Work out the finished part from the listing and answer in its coordinate system (mm). A direction names the side the tool comes from. Round coordinates to 2 decimals unless told otherwise and drop trailing zeros. Order: outer loops, then holes, each group sorted by start corner. A loop starts at its lowest first (then second) coordinate and runs counter-clockwise, first axis right, second up.
from build123d import *

# Parameters (mm, degrees)
SKETCH1_R               = 16.63
SKETCH1_R_2             = 4.8
SKETCH1_R_3             = 2.625
BOSS_EXTRUDE2_DEPTH     = 2
SKETCH5_R               = 6.625
SKETCH5_R_2             = 2.625
BOSS_EXTRUDE3_DEPTH     = 8
SKETCH4_R               = 1.6
CUT_EXTRUDE1_DEPTH      = 8
CIRPATTERN1_COUNT       = 2
CUT_EXTRUDE2_DEPTH      = 10
CUT_EXTRUDE2_DEPTH_BACK = 8
SKETCH6_R               = 1.5


with BuildPart() as part:
    # Sketch1 → Boss-Extrude2 (new body)
    # profile 1 of 2: a face of its own
    with BuildSketch(Plane(origin=(0, 0, 0), x_dir=(1, 0, 0), z_dir=(0, 1, 0))):
        with Locations(Location((0, 0, 0), (0, 0, 270))):
            Circle(SKETCH1_R)
        Circle(SKETCH1_R_2, mode=Mode.SUBTRACT)
    # profile 2 of 2: a face of its own
    with BuildSketch(Plane(origin=(0, 0, 0), x_dir=(1, 0, 0), z_dir=(0, 1, 0))):
        Circle(SKETCH1_R_2)
        with Locations(Location((0, 0, 0), (0, 0, 270))):
            Circle(SKETCH1_R_3, mode=Mode.SUBTRACT)
    extrude(amount=BOSS_EXTRUDE2_DEPTH)

    # Sketch5 → Boss-Extrude3 (add)
    with BuildSketch(Plane(origin=(0, 2, 0), x_dir=(1, 0, 0), z_dir=(0, 1, 0))):
        with Locations(Location((0, 0, 0), (0, 0, 270))):
            Circle(SKETCH5_R)
        with Locations(Location((0, 0, 0), (0, 0, 270))):
            Circle(SKETCH5_R_2, mode=Mode.SUBTRACT)
    extrude(amount=BOSS_EXTRUDE3_DEPTH)

    # Sketch4 → Cut-Extrude1 (cut)
    with BuildSketch(Plane(origin=(0, 2, 0), x_dir=(1, 0, 0), z_dir=(0, 1, 0))):
        with Locations(Location((11.625, 0, 0), (0, 0, 270))):
            Circle(SKETCH4_R)
    cut_extrude1 = extrude(amount=-CUT_EXTRUDE1_DEPTH, mode=Mode.SUBTRACT)

    # CirPattern1: Cut-Extrude1 ×2 about axis
    cirpattern1_axis = Axis((0, 0, 0), (0, 1, 0))
    for i in range(1, CIRPATTERN1_COUNT):
        add(cut_extrude1.rotate(cirpattern1_axis, i * 360 / CIRPATTERN1_COUNT), mode=Mode.SUBTRACT)

    # Sketch6 → Cut-Extrude2 (cut, two sides: drawn at the far end of the back side and taken through both)
    with BuildSketch(Plane(origin=(0, 0, 0), x_dir=(0, 0, -1), z_dir=(1, 0, 0)).offset(-CUT_EXTRUDE2_DEPTH_BACK)):
        with Locations(Location((0, 5.866356901, 0), (0, 0, 180))):
            Circle(SKETCH6_R)
    extrude(amount=CUT_EXTRUDE2_DEPTH + CUT_EXTRUDE2_DEPTH_BACK, mode=Mode.SUBTRACT)


solid = part.part
Item 1: Find section B-B (x = 0). Write down the section's boundary in (y, z) (3 decimals).
Item 2: Find the intervals of material crossed by line 1 along X through (y, z) = (0.7, 0) (3 decimals); line 2 along Y through (x, z) = (-5.5, -13.5); line 3 along Z through (x, y) = (-0.5, 9.25), in increasing order.
Item 3: Find section A-A (z = 0). Write down the section's boundary in (x, y) (3 decimals), plus the area to 3 significant figures.
Item 4: Given pin 1 (2.5 mm diameter, centred on y = 5.87, z = 0, fed in from +X); pin 2 (3 mm diameter, centred on y = 8.5, z = -7, fed in from -X); pin 3 (1.5 mm diameter, centred on x = 5, y = 3.5, fed in from -Z); pin 4 (2 mm diameter, centred on x = -5, z = 11, fed in from +Y), each flat-ended and moving along its own axis, determine where each tip first touches the part or whether it passes through.
Item 5: Find section C-C (y = 8). Write down the section's boundary in (x, z) (3 decimals), plus the area to 3 significant figures.
Item 6: A tool of negligible diameter and unlimited length cuts with its end or side. For faces 1 (the face through (4.36, 7.33, -0.33)), 2 (the face through (0, 2, 7)), from which of +Z, -Z, +X, -X, +Y, -Y can it reach the whole face along a straight path? Write none if from no direction.
Item 7: Find section D-D (x = -3.5). Write down the section's boundary in (y, z) (3 decimals).
Item 8: For a pull along Y with two mould halves and no side action, classify faces 3 (the face through (-4.4, 5.8, -1.5)), 4 (the face through (-16.235, 0.986, -3.605)), 5 (the face through (0, 10, 3)), 6 (the face through (0, 0, 3)) as released by +Y, released by -Y, zero draft, split by the parting line, or undercut.
Model answer:
1. outline: (0, -16.63) - (2, -16.63) - (2, -6.625) - (10, -6.625) - (10, -2.625) - (0, -2.625) - close; (0, 2.625) - (10, 2.625) - (10, 6.625) - (2, 6.625) - (2, 16.63) - (0, 16.63) - close
2. line 1: x = -16.63 to -13.225, -10.025 to -2.625, 2.625 to 10.025, 13.225 to 16.63
2. line 2: y = 0 to 2
2. line 3: z = -6.61 to -2.58, 2.58 to 6.61
3. outline: (-16.63, 0) - (-13.225, 0) - (-13.225, 2) - (-16.63, 2) - close; (-10.025, 0) - (-2.625, 0) - (-2.625, 4.366) - (-6.625, 4.366) - (-6.625, 2) - (-10.025, 2) - close; (-6.625, 7.366) - (-2.625, 7.366) - (-2.625, 10) - (-6.625, 10) - close; (2.625, 0) - (10.025, 0) - (10.025, 2) - (6.625, 2) - (6.625, 4.366) - (2.625, 4.366) - close; (2.625, 7.366) - (6.625, 7.366) - (6.625, 10) - (2.625, 10) - close; (13.225, 0) - (16.63, 0) - (16.63, 2) - (13.225, 2) - close
3. area: 83.2 mm2
4. pin 1: passes through
4. pin 2: stops at x = -3.69
4. pin 3: stops at z = -5.08
4. pin 4: stops at y = 2
5. outline: circle Ø13.25 at (0, 0); hole circle Ø5.25 at (0, 0)
5. area: 116 mm2
6. face 1: +X, -X
6. face 2: +Y
7. outline: (0, -16.258) - (2, -16.258) - (2, -5.625) - (10, -5.625) - (10, 5.625) - (2, 5.625) - (2, 16.258) - (0, 16.258) - close; hole circle Ø3 at (5.866, 0)
8. face 3: undercut
8. face 4: zero draft
8. face 5: released by +Y
8. face 6: released by -Y
